The model under review builds one solid part; all positions refer to its coordinate system, in mm. Face numbers are marked on the shaded views. A direction names the side the tool comes from. Give positions to 0.01 mm unless a question says otherwise; leave off trailing zeros. Loops run counter-clockwise (first coordinate to the right, second up) from the corner with the lowest first, then second, coordinate; pieces in that order, holes last. Notation, with made-up numbers: (10, -1) - (46, -1) arc R18 ccw to (46, 22) - close; hole circle Ø2 at (1, 81.25). An arc over 180 degrees is marked (long way). Return JSON: item names as keys, results as strings. Group by question number.
```python
from build123d import *

# Parameters (mm, degrees)
SKETCH_1_W          = 60
SKETCH_1_H          = 56
EXTRUDE_1_DEPTH     = 20
EXTRUDE_START       = -15
SKETCH_6_W          = 30
SKETCH_6_H          = 15
EXTRUDE_3_DEPTH     = 5
SKETCH_7_R          = 1.5
CUT_EXTRUDE_2_DEPTH = 70.166465863
CUT_EXTRUDE_START   = -15
SKETCH_8_R          = 2.75
CUT_EXTRUDE_3_DEPTH = 5
FILLET_2_R          = 4
SKETCH_9_W          = 45
SKETCH_9_H          = 35
CUT_EXTRUDE_4_DEPTH = 70.166465863
FILLET_3_R          = 4


with BuildPart() as part:
    # 草图1 → 凸台-拉伸1 (new body)
    with BuildSketch(Plane(origin=(0, 0, 0), x_dir=(0, 0, -1), z_dir=(1, 0, 0))):
        Rectangle(SKETCH_1_W, SKETCH_1_H)
    extrude(amount=EXTRUDE_1_DEPTH)

    # 草图6 → 凸台-拉伸3 (add)
    with BuildSketch(Plane(origin=(20, 0, 0), x_dir=(0, 0, -1), z_dir=(1, 0, 0)).offset(EXTRUDE_START)):
        with Locations((45, -2.5)):
            Rectangle(SKETCH_6_W, SKETCH_6_H)
        with Locations((-45, -2.5)):
            Rectangle(SKETCH_6_W, SKETCH_6_H)
    extrude(amount=-EXTRUDE_3_DEPTH)

    # 草图7 → 切除-拉伸2 (cut, through all)
    with BuildSketch(Plane(origin=(20, 0, 0), x_dir=(0, 0, -1), z_dir=(1, 0, 0))):
        with Locations((-13, 24.75)):
            Circle(SKETCH_7_R)
        with Locations((13, 24.75)):
            Circle(SKETCH_7_R)
        with Locations((13, -24.75)):
            Circle(SKETCH_7_R)
        with Locations((-13, -24.75)):
            Circle(SKETCH_7_R)
    extrude(amount=-CUT_EXTRUDE_2_DEPTH, mode=Mode.SUBTRACT)

    # 草图8 → 切除-拉伸3 (cut)
    with BuildSketch(Plane(origin=(20, 0, 0), x_dir=(0, 0, -1), z_dir=(1, 0, 0)).offset(CUT_EXTRUDE_START)):
        with Locations((-50.5, -3)):
            Circle(SKETCH_8_R)
        with Locations((50.5, -3)):
            Circle(SKETCH_8_R)
    extrude(amount=-CUT_EXTRUDE_3_DEPTH, mode=Mode.SUBTRACT)

    # 圆角2
    fillet_2_edges = [part.edges().sort_by_distance(p)[0] for p in [
        (2.5, 5, -60),
        (2.5, -10, -60),
        (2.5, -10, 60),
        (2.5, 5, 60),
        (10, 28, 30),
        (10, 28, -30),
        (10, -28, -30),
        (10, -28, 30),
    ]]
    fillet(fillet_2_edges, radius=FILLET_2_R)

    # 草图9 → 切除-拉伸4 (cut, through all)
    with BuildSketch(Plane(origin=(20, 0, 0), x_dir=(0, 0, -1), z_dir=(1, 0, 0))):
        Rectangle(SKETCH_9_W, SKETCH_9_H)
    extrude(amount=-CUT_EXTRUDE_4_DEPTH, mode=Mode.SUBTRACT)

    # 圆角3
    fillet_3_edges = [part.edges().sort_by_distance(p)[0] for p in [
        (10, -17.5, 22.5),
        (10, 17.5, 22.5),
        (10, 17.5, -22.5),
        (10, -17.5, -22.5),
    ]]
    fillet(fillet_3_edges, radius=FILLET_3_R)


solid = part.part
```
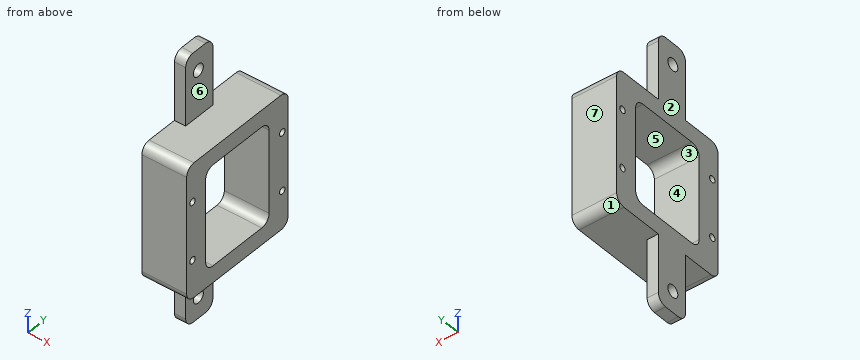
1) To check wall thickness, follow line 1 (Y direction, x = 13.25, z = 13); line 2 (Z direction, x = 7.75, y = -3); line 3 (Y direction, x = 18, z = 0). State the ranges of each line that lie inside material, in increasing order.
2) We need section D-D, the plane x = 3.5. Count the separate pieces of the cut face and the enclosed holes in it, plus the area to 3 significant figures.
3) Draft analysis for pull direction Z (two halves, no side actions). For the marked faces 1, 2, 3 and 4, state which applies: +Z half, -Z half, draft (parallel to the pull), parting line (faces both ways), or undercut.
4) We need section C-C, the plane z = 13. Write out the cut boundary in (x, y), plus the area to 3 significant figures.
5) Tool access review of the marked faces 5, 6 and 7: name each direction out of +Z, -Z, +X, -X, +Y, -Y from which nothing blocks a thin tool from reaching the whole face with its end or side.
6) We need section A-A, the plane y = -3. Write out the cut boundary in (x, z).
7) We need section B-B, the plane x = 15.75. Write out the cut boundary in (y, z).
8) For pin 1 Ø16.5 at (y, z) = (-0.5, 45) entering from +X; pin 2 Ø10 at (x, y) = (14.5, -20) entering from -Z; pin 3 Ø4 at (x, z) = (2, 45.5) entering from -Y, all flat-tipped, find the tip position at first contact; note any pin that passes through.
Findings:
{
 "1": {"line 1": "y = -28 to -26.25, -23.25 to -17.5, 17.5 to 23.25, 26.25 to 28", "line 2": "z = -30 to -22.5, 22.5 to 30", "line 3": "y = -28 to -17.5, 17.5 to 28"},
 "2": {"separate pieces": "1", "enclosed holes": "7", "area": "2,600 mm^2"},
 "3": {"face 1": "-Z half", "face 2": "draft", "face 3": "undercut", "face 4": "undercut"},
 "4": {"outline": "(0, -28) - (20, -28) - (20, -26.25) - (0, -26.25) - close; (0, -23.25) - (20, -23.25) - (20, -17.5) - (0, -17.5) - close; (0, 17.5) - (20, 17.5) - (20, 23.25) - (0, 23.25) - close; (0, 26.25) - (20, 26.25) - (20, 28) - (0, 28) - close", "area": "300 mm^2"},
 "5": {"face 5": "+X, -X", "face 6": "+Z, +X, +Y, -Y", "face 7": "+Z, -Z, +X, -X, +Y"},
 "6": {"outline": "(0, -60) - (5, -60) - (5, -53.25) - (0, -53.25) - close; (0, -47.75) - (5, -47.75) - (5, -30) - (20, -30) - (20, -22.5) - (0, -22.5) - close; (0, 22.5) - (20, 22.5) - (20, 30) - (5, 30) - (5, 47.75) - (0, 47.75) - close; (0, 53.25) - (5, 53.25) - (5, 60) - (0, 60) - close"},
 "7": {"outline": "(-28, -26) arc R4 ccw to (-24, -30) - (24, -30) arc R4 ccw to (28, -26) - (28, 26) arc R4 ccw to (24, 30) - (-24, 30) arc R4 ccw to (-28, 26) - close; hole circle Ø3 at (-24.75, -13); hole circle Ø3 at (-24.75, 13); hole (-17.5, -18.5) arc R4 ccw to (-13.5, -22.5) - (13.5, -22.5) arc R4 ccw to (17.5, -18.5) - (17.5, 18.5) arc R4 ccw to (13.5, 22.5) - (-13.5, 22.5) arc R4 ccw to (-17.5, 18.5) - close; hole circle Ø3 at (24.75, -13); hole circle Ø3 at (24.75, 13)"},
 "8": {"pin 1": "stops at x = 5", "pin 2": "stops at z = -30", "pin 3": "stops at y = -10"}
}
